Could you check a few things on this model? Use its own coordinates, in mm. A direction names the side the tool comes from. Round coordinates to 2 decimals unless told otherwise and drop trailing zeros. Loops run counter-clockwise (first coordinate to the right, second up) from the corner with the lowest first, then second, coordinate; pieces in that order, holes last.
from build123d import *

# Parameters (mm, degrees)
BOSS_EXTRUDE1_DEPTH = 55
SKETCH2_W           = 15
SKETCH2_H           = 50.876134921
CUT_EXTRUDE1_DEPTH  = 2.6
SKETCH3_R           = 2.1
CUT_EXTRUDE2_DEPTH  = 32.6
FILLET2_R           = 6
SKETCH4_R           = 3.65
CUT_EXTRUDE3_DEPTH  = 22.6


with BuildPart() as part:
    # Sketch1 → Boss-Extrude1 (new body)
    with BuildSketch(Plane.XY):
        with BuildLine():
            Line((-10.5, 16.441414071), (-10.5, -34.43472085))
            ThreePointArc((-10.5, -34.43472085), (-33.154419012, -14.027989876), (-32.026237733, 16.441414071))
            Line((-32.026237733, 16.441414071), (-10.5, 16.441414071))
        make_face()
    extrude(amount=BOSS_EXTRUDE1_DEPTH)

    # Sketch2 → Cut-Extrude1 (cut)
    with BuildSketch(Plane(origin=(-10.5, 0, 0), x_dir=(0, 0, -1), z_dir=(1, 0, 0))):
        with Locations((-47.5, -8.99665339)):
            Rectangle(SKETCH2_W, SKETCH2_H)
    extrude(amount=-CUT_EXTRUDE1_DEPTH, mode=Mode.SUBTRACT)

    # Sketch3 → Cut-Extrude2 (cut)
    with BuildSketch(Plane(origin=(-10.5, 0, 0), x_dir=(0, 0, -1), z_dir=(1, 0, 0))):
        with Locations((-8, 4.681414071)):
            Circle(SKETCH3_R)
        with Locations((-24, 4.681414071)):
            Circle(SKETCH3_R)
        with Locations((-24, -19.318585929)):
            Circle(SKETCH3_R)
        with Locations((-8, -19.318585929)):
            Circle(SKETCH3_R)
    extrude(amount=-CUT_EXTRUDE2_DEPTH, mode=Mode.SUBTRACT)

    # Fillet2
    fillet2_edges = [part.edges().sort_by_distance(p)[0] for p in [
        (-33.666422287, -12.750372951, 55),
        (-32.026237733, 16.441414071, 27.5),
    ]]
    fillet(fillet2_edges, radius=FILLET2_R)

    # Sketch4 → Cut-Extrude3 (cut)
    with BuildSketch(Plane.ZY.offset(36)):
        with Locations((8, 4.681414071)):
            Circle(SKETCH4_R)
        with Locations((24, 4.681414071)):
            Circle(SKETCH4_R)
        with Locations((24, -19.318585929)):
            Circle(SKETCH4_R)
        with Locations((8, -19.318585929)):
            Circle(SKETCH4_R)
    extrude(amount=-CUT_EXTRUDE3_DEPTH, mode=Mode.SUBTRACT)


solid = part.part
Item 1: If we section it at C-C, the plane z = 45: Please give me the cut outline in (x, y), then the cut area to 3 significant figures.
Results list:
outline: (-33.75, 12.53) arc R36 ccw to (-13.1, -33.53) - (-13.1, 16.44) - (-28.12, 16.44) arc R6 ccw to start
area: 909 mm2
Item 2: We'd pull the mould along Z, two halves only. Please class faces 1 (the flat face through (-20, -3, 0)), 2 (the cylindrical face through (-24.85, 7.76, 9.96)), 3 (the flat face through (-12, -9, 40)): released by +Z, released by -Z, zero draft, split by the parting line, or undercut.
Results list:
face 1: released by -Z
face 2: undercut
face 3: released by +Z
Item 3: If we section it at A-A, the plane z = 24: Please give me the cut outline in (x, y), then the cut area to 3 significant figures.
Results list:
outline: (-35.99, 1.03) arc R36 ccw to (-32.41, -15.67) - (-13.4, -15.67) - (-13.4, -17.22) - (-10.5, -17.22) - (-10.5, 2.58) - (-13.4, 2.58) - (-13.4, 1.03) - close; (-35.02, 8.33) - (-13.4, 8.33) - (-13.4, 6.78) - (-10.5, 6.78) - (-10.5, 16.44) - (-28.12, 16.44) arc R6 ccw to (-33.75, 12.53) arc R36 ccw to start; (-27.72, -22.97) arc R36 ccw to (-10.5, -34.43) - (-10.5, -21.42) - (-13.4, -21.42) - (-13.4, -22.97) - close
area: 731 mm2
Item 4: For faces 4 (the flat face through (-13.4, 3, 26)), 5 (the cylindrical face through (-31.5, 15.4, 27.6)), which set-ups out of +Z, -Z, +X, -X, +Y, -Y let a thin tool reach every point of the face, with its end or its side?
Results list:
face 4: -X
face 5: +Z, -Z, -X, +Y
Item 5: Will these pins go through, and if not, where does the flat tip stop? pin 1 (3.5 mm diameter, centred on y = -19.32, z = 8, fed in from +X); pin 2 (5.5 mm diameter, centred on y = 4.68, z = 8, fed in from -X); pin 3 (4.5 mm diameter, centred on y = -15.5, z = 46, fed in from +X); pin 4 (1.5 mm diameter, centred on y = -4.5, z = 10, fed in from -X).
Results list:
pin 1: passes through
pin 2: stops at x = -13.4
pin 3: stops at x = -13.1
pin 4: stops at x = -35.8
Item 6: If I drill on line 1 along Y through (x, z) = (-19.75, 8); line 2 along Y through (x, z) = (-26.5, 8); line 3 along X through (y, z) = (5, 21), over which ranges is the centre line in solid material (lowest first)?
Results list:
line 1: y = -30.1 to -22.97, -15.67 to 1.03, 8.33 to 16.44
line 2: y = -24.37 to -22.97, -15.67 to 1.03, 8.33 to 16.44
line 3: x = -13.4 to -10.5
Item 7: If we section it at B-B, the plane y = 5.5: Count the separate pieces of the cut face and the enclosed holes in it, then the cut area to 3 significant figures.
Results list:
separate pieces: 3
enclosed holes: 0
area: 994 mm2
